Can you work these out from the model? Positions are in its coordinate system, mm. A direction names the side the tool comes from. Give positions to 0.01 mm unless a question says otherwise; leave off trailing zeros. Order: outer loops, then holes, each group sorted by start corner. A loop starts at its lowest first (then second) coordinate and runs counter-clockwise, first axis right, second up. Notation, with made-up numbers: M -36,-5 L 12,-5 A30 ccw 12,34 Z; hole C 48,-20.5 d3. An arc over 180 degrees is marked long. Answer as a JSON object with one key per item and string values.
Autodesk Inventor part; units mm, degrees
ref_plane "作業平面1" through (0, 3.5, 0) normal (0, 1, 0) x (1, 0, 0)
ref_plane "YZ Plane" through (0, 0, 0) normal (1, 0, 0) x (0, 1, 0)
ref_plane "XZ Plane" through (0, 0, 0) normal (0, 1, 0) x (-1, 0, 0)
sketch "スケッチ1" plane through (0, 0, 0) normal (0, 1, 0) x (-1, 0, 0)
  circle A0 centre (0, 0) radius 5
  circle A1 centre (0, 0) radius 3.1
  dimension "d0" = 10
  dimension "d8" = 6.2
extrude "押し出し1" add sketch "スケッチ1" along normal blind 7
ref_plane "作業平面1" through (0, 3.5, 0) normal (0, 1, 0) x (1, 0, 0)
sketch "スケッチ5" plane through (0, 3.5, 0) normal (0, 1, 0) x (1, 0, 0)
  circle A0 centre (0, 0) radius 1.75
  circle A1 centre (0, 0) radius 3.1
  dimension "d9" = 3.5
extrude "押し出し4" add sketch "スケッチ5" along normal mid plane 3
properties part number "belt_roller_outside"
1) Thinking about a two-plate mould opening in Z: for faces 1 (the face through (1.08, 3.45, 4.88)), 2 (the face through (-3.3, 0, 0.1)), 3 (the face through (2, 2, 0)), which applies, pulls with the +Z half, pulls with the -Z half, needs draft (parallel to the pull), parting line crosses it, or undercut?
Results found:
{"face 1": "parting line crosses it", "face 2": "needs draft", "face 3": "undercut"}
2) I'm going to push flat-ended pins straight in: pin 1 Ø3 at (x, z) = (0, 0) entering from -Y; pin 2 Ø1 at (x, y) = (0.5, 1) entering from -Z; pin 3 Ø4 at (y, z) = (6, -3) entering from -X; pin 4 Ø1.9 at (x, z) = (-1, 1) entering from +Y. Where does each tip first touch, or does it pass through?
Results found:
{"pin 1": "passes through", "pin 2": "stops at z = -5", "pin 3": "stops at x = -4.9", "pin 4": "stops at y = 5"}
3) I want a section at D-D on x = 4. Write out the boundary of the cut face in (y, z), and give its area (3 significant figures).
Results found:
{"outline": "M 0,-3 L 7,-3 L 7,3 L 0,3 Z", "area": "42.0 mm²"}
4) For faces 4 (the face through (-3.3, 7, 0.1)), 5 (the face through (-1.43, 0.99, 2.75)), 6 (the face through (2, 5, 0)), which set-ups out of +Z, -Z, +X, -X, +Y, -Y let a thin tool reach every point of the face, with its end or its side?
Results found:
{"face 4": "+Z, -Z, +X, -X, +Y", "face 5": "-Y", "face 6": "+Y"}
5) I want a section at C-C on y = 6.75. Write out the boundary of the cut face in (x, z), and give its area (3 significant figures).
Results found:
{"outline": "C 0,0 d10; hole C 0,0 d6.2", "area": "48.3 mm²"}
6) I want a section at B-B on z = 0. Write out the boundary of the cut face in (x, y).
Results found:
{"outline": "M -5,0 L -3.1,0 L -3.1,2 L -1.75,2 L -1.75,5 L -3.1,5 L -3.1,7 L -5,7 Z; M 1.75,2 L 3.1,2 L 3.1,0 L 5,0 L 5,7 L 3.1,7 L 3.1,5 L 1.75,5 Z"}
7) I need wall thicknesses on L1, parallel to Z at x = 0, y = 4.2; L2, parallel to Z at x = 0, y = 0.85; L3, parallel to Y at x = 1.75, z = 2.5. Which ranges of each line are inside material? Lowest first, please.
Results found:
{"L1": "z = -5 to -1.75, 1.75 to 5", "L2": "z = -5 to -3.1, 3.1 to 5", "L3": "y = 2 to 5"}
8) I want a section at A-A on x = 0. Write out the boundary of the cut face in (y, z).
Results found:
{"outline": "M 0,-5 L 7,-5 L 7,-3.1 L 5,-3.1 L 5,-1.75 L 2,-1.75 L 2,-3.1 L 0,-3.1 Z; M 0,3.1 L 2,3.1 L 2,1.75 L 5,1.75 L 5,3.1 L 7,3.1 L 7,5 L 0,5 Z"}
